Source: CAD feature listing. Evaluate the final solid. Frame: model axes, mm. A direction names the side the tool comes from. Coordinates: 2 decimals unless noted, no trailing zeros. Write each loop counter-clockwise with the first axis right and the second up, starting at its lowest first coordinate (ties: lowest second). Pieces come first, ordered by that corner, then holes. Notation, with made-up numbers: (54, 76) - (84, 76) arc R24 cw to (84, 88) - close; hole circle Ø8 at (78.5, 34). An arc over 180 degrees is marked (long way). One line per item, written item: value.
from build123d import *

# Parameters (mm, degrees)
CROQUIS1_R              = 6.35
CROQUIS1_R_2            = 4
SALIENTE_EXTRUIR1_DEPTH = 10
CROQUIS2_W              = 6
CROQUIS2_H              = 1


with BuildPart() as part:
    # Croquis1 → Saliente-Extruir1 (new body)
    with BuildSketch(Plane.XY):
        Circle(CROQUIS1_R)
        Circle(CROQUIS1_R_2, mode=Mode.SUBTRACT)
    extrude(amount=SALIENTE_EXTRUIR1_DEPTH)

    # Croquis2 → Cortar-Revolución1 (revolve, cut)
    with BuildSketch(Plane(origin=(0, 0, 0), x_dir=(0, 0, -1), z_dir=(1, 0, 0))):
        with Locations((-5, 5.85)):
            Rectangle(CROQUIS2_W, CROQUIS2_H)
    revolve(axis=Axis((0, 0, 10), (0, 0, -1)), mode=Mode.SUBTRACT)


solid = part.part
1) Section query A-A on x = 0. Output: boundary loops of the cut face in (y, z).
Values found:
outline: (-6.35, 0) - (-4, 0) - (-4, 10) - (-6.35, 10) - (-6.35, 8) - (-5.35, 8) - (-5.35, 2) - (-6.35, 2) - close; (4, 0) - (6.35, 0) - (6.35, 2) - (5.35, 2) - (5.35, 8) - (6.35, 8) - (6.35, 10) - (4, 10) - close
2) Section query C-C on z = 6. Output: boundary loops of the cut face in (x, y).
Values found:
outline: circle Ø10.7 at (0, 0); hole circle Ø8 at (0, 0)
3) Reachability of faces 4 (the flat face through (-5, 3, 2)), 5 (the cylindrical face through (6.057, 1.907, 0.986)) from +Z, -Z, +X, -X, +Y, -Y: full face, straight path, thin tool, end or side. Return the list, or none.
Values found:
face 4: none
face 5: +Z, -Z
4) Draft query along Z for faces 1 (the cylindrical face through (-5.223, -1.16, 4.958)), 2 (the flat face through (1.3, -4.1, 0)), 3 (the flat face through (1.3, -4.1, 10)). Return one class per face: released by +Z, released by -Z, zero draft, split by the parting line, or undercut.
Values found:
face 1: undercut
face 2: released by -Z
face 3: released by +Z
5) Contact query for flat-ended pins moving along their axis: P1, Ø2, axis at y = -0.5, z = 6, coming from the -X side; P2, Ø6, axis at x = -3, z = 3, coming from the -Y side; P3, Ø3, axis at y = -3, z = 3, coming from the -X side; P4, Ø1, axis at x = 0, y = 2.5, coming from the -Z side. Output: stop coordinate, or through.
Values found:
P1: x = -5.35
P2: y = -6.35
P3: x = -6.06
P4: through
6) Material intervals for line 1 (Z direction, x = 5, y = 2); line 2 (X direction, y = 3, z = 4.5); line 3 (Y direction, x = 1, z = 5.5), sorted ascending.
Values found:
line 1: 0 to 2, 8 to 10
line 2: -4.43 to -2.65, 2.65 to 4.43
line 3: -5.26 to -3.87, 3.87 to 5.26
